Part print with two shaded views. Sizes in mm from the minimum x, y, z corner. A direction names the side the tool comes from. Coordinates: 2 decimals unless noted, no trailing zeros. Write each loop counter-clockwise with the first axis right and the second up, starting at its lowest first coordinate (ties: lowest second). Pieces come first, ordered by that corner, then holes.
Q1. Band-saw the part on B-B, the plane y = 14. Write the cut outline in (x, z).
Q2. Band-saw the part on C-C, the plane x = 115.5. Write the cut outline in (y, z).
Q3. Pin check, flat tip, straight feed: P1, Ø5, axis at x = 20.5, z = 20.5, coming from the +Y side. Stop position of the tip, or through.
Q4. Drill centre lines: probe 1 along Z at (x, y) = (142, 44); probe 2 along Y at (x, z) = (56, 116). Where is each one in solid material? Low to high.
Q5. Pull direction X, two halves, no side cores. Call the marked faces 3, 4, 5 and 6: released by +X, released by -X, zero draft, split by the parting line, or undercut.
Q6. Band-saw the part on A-A, the plane z = 129. Write the cut outline in (x, y), plus the area to 3 significant figures.
Q7. Which spindle directions (+Z, -Z, +X, -X, +Y, -Y) get a long thin tool onto all of the face, cutting with end or side? Do the marked faces 1 and 2. Say none if no direction does.
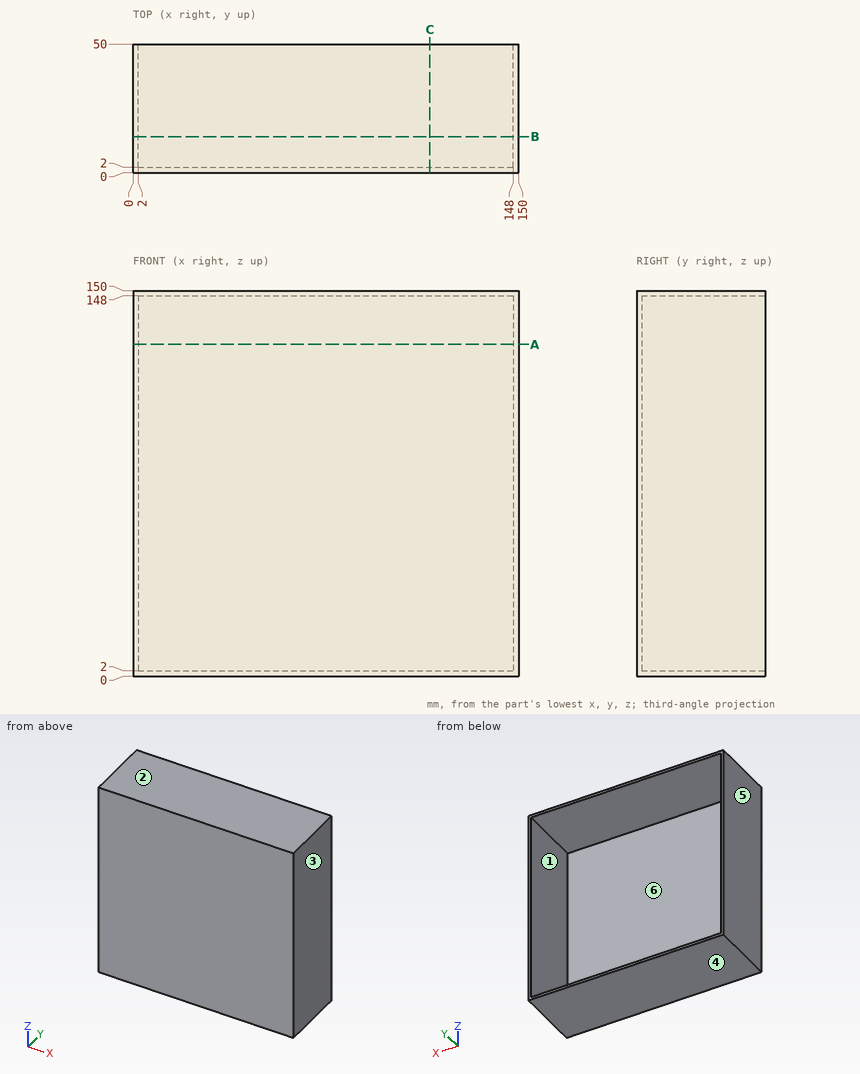
Answer sheet:
1. outline: (0, 0) - (150, 0) - (150, 150) - (0, 150) - close; hole (2, 2) - (148, 2) - (148, 148) - (2, 148) - close
2. outline: (0, 0) - (50, 0) - (50, 2) - (2, 2) - (2, 148) - (50, 148) - (50, 150) - (0, 150) - close
3. P1: stops at y = 2
4. probe 1: z = 0 to 2, 148 to 150
4. probe 2: y = 0 to 2
5. face 3: released by +X
5. face 4: zero draft
5. face 5: released by -X
5. face 6: undercut
6. outline: (0, 0) - (150, 0) - (150, 50) - (148, 50) - (148, 2) - (2, 2) - (2, 50) - (0, 50) - close
6. area: 492 mm2
7. face 1: +Y
7. face 2: +Z, +X, -X, +Y, -Y
